The listing builds one solid part. Answer for the finished solid, in the listing's coordinates (mm). Face numbers are marked on the shaded views. A direction names the side the tool comes from. Give positions to 0.01 mm unless a question says otherwise; leave off trailing zeros. Loops run counter-clockwise (first coordinate to the right, second up) from the corner with the lowest first, then second, coordinate; pieces in that order, holes last. Notation, with made-up numbers: (-28.5, -20.5) - (-21.5, -20.5) arc R25 cw to (-21.5, 15.5) - close; hole circle Ø2 at (16.25, -6). An arc over 180 degrees is marked (long way). Answer as CSV lines item,"result". Start each with the question number.
1) A cutting plane is placed at A-A (z = 0). Determine the outline of the cut face in (x, y).
2) For the marked faces 4 and 5, determine the directions among +Z, -Z, +X, -X, +Y, -Y from which every point of the face is accessible in a straight line to the end or side of a thin tool.
3) A cutting plane is placed at D-D (x = 6.5). Determine the outline of the cut face in (y, z).
4) Find the intervals of material crossed by line 1 along Z through (x, y) = (-5.75, 8.25); line 2 along Z through (x, y) = (0, 6), in increasing order.
5) Flat-ended cylindrical pins translate along their axes: pin 1 (0.5 mm diameter, centred on y = 9, z = -7.5, fed in from -X); pin 2 (1.5 mm diameter, centred on x = -1.5, y = 8, fed in from +Z); pin 3 (0.6 mm diameter, centred on x = 0.5, z = -9, fed in from +Y); pin 4 (11 mm diameter, centred on x = 0, z = 0, fed in from +Y). Find the tip coordinate at first contact, or state that the pin passes through.
6) A cutting plane is placed at B-B (x = 0). Determine the outline of the cut face in (y, z).
7) For a pull along X with two mould halves and no side action, classify the marked faces 1, 2 and 3 as pulls with the +X half, pulls with the -X half, needs draft (parallel to the pull), parting line crosses it, or undercut.
```python
from build123d import *

# Parameters (mm, degrees)
SKETCH1_R           = 9.2
BOSS_EXTRUDE1_DEPTH = 8.2
BOSS_EXTRUDE2_DEPTH = 1.8


with BuildPart() as part:
    # Sketch1 → Boss-Extrude1 (new body)
    with BuildSketch(Plane(origin=(0, 0, 0), x_dir=(1, 0, 0), z_dir=(0, 1, 0))):
        Polygon((-10.1, 10.1), (-7, 10.1), (-7.5, 8.7), (-4.5, 8.7), (-5, 10.1), (5, 10.1), (4.5, 8.7), (7.5, 8.7), (7, 10.1), (10.1, 10.1), (10.1, 6.5), (10.1, 4.5), (10.1, -4.5), (10.1, -6.5), (10.1, -10.1), (7, -10.1), (7.5, -11.5), (4.5, -11.5), (5, -10.1), (-5, -10.1), (-4.5, -11.5), (-7.5, -11.5), (-7, -10.1), (-10.1, -10.1), (-10.1, -6.5), (-11.5, -7), (-11.5, -4), (-10.1, -4.5), (-10.1, 4.5), (-11.5, 4), (-11.5, 7), (-10.1, 6.5), align=None)
        with Locations(Location((0, 0, 0), (0, 0, 270))):
            Circle(SKETCH1_R, mode=Mode.SUBTRACT)
    extrude(amount=BOSS_EXTRUDE1_DEPTH)

    # Sketch2 → Boss-Extrude2 (add)
    with BuildSketch(Plane(origin=(0, 8.2, 0), x_dir=(1, 0, 0), z_dir=(0, 1, 0))):
        with BuildLine():
            Line((-4.1, 10.1), (-4.1, 5.1))
            ThreePointArc((-4.1, 5.1), (-4.392893219, 4.392893219), (-5.1, 4.1))
            Line((-5.1, 4.1), (-10.1, 4.1))
            Line((-10.1, 4.1), (-10.1, 10.1))
            Line((-10.1, 10.1), (-4.1, 10.1))
        make_face()
        with BuildLine():
            Line((10.1, 4.1), (10.1, 10.1))
            Line((10.1, 10.1), (4.1, 10.1))
            Line((4.1, 10.1), (4.1, 5.1))
            ThreePointArc((4.1, 5.1), (4.392893219, 4.392893219), (5.1, 4.1))
            Line((5.1, 4.1), (10.1, 4.1))
        make_face()
        with BuildLine():
            Line((4.1, -10.1), (4.1, -5.1))
            ThreePointArc((4.1, -5.1), (4.392893219, -4.392893219), (5.1, -4.1))
            Line((5.1, -4.1), (10.1, -4.1))
            Line((10.1, -4.1), (10.1, -10.1))
            Line((10.1, -10.1), (4.1, -10.1))
        make_face()
        with BuildLine():
            Line((-10.1, -4.1), (-10.1, -10.1))
            Line((-10.1, -10.1), (-4.1, -10.1))
            Line((-4.1, -10.1), (-4.1, -5.1))
            ThreePointArc((-4.1, -5.1), (-4.392893219, -4.392893219), (-5.1, -4.1))
            Line((-5.1, -4.1), (-10.1, -4.1))
        make_face()
    extrude(amount=BOSS_EXTRUDE2_DEPTH)


solid = part.part
```
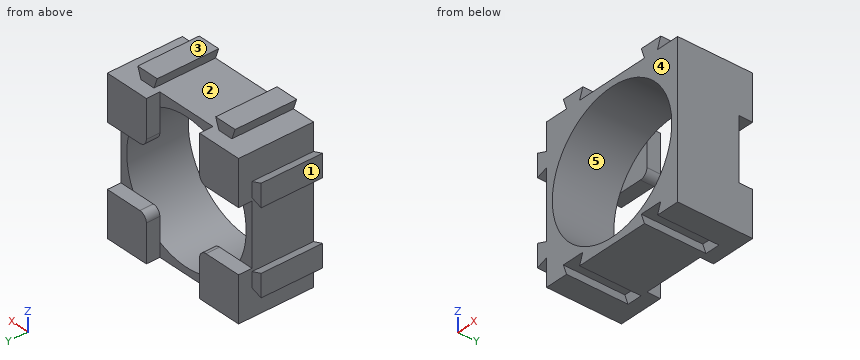
Ans:
1,outline,"(-10.1, 0) - (-9.2, 0) - (-9.2, 8.2) - (-10.1, 8.2) - close; (9.2, 0) - (10.1, 0) - (10.1, 8.2) - (9.2, 8.2) - close"
2,face 4,"+Z, -Z, +X, -X, -Y"
2,face 5,"-Y"
3,outline,"(0, -8.7) - (8.2, -8.7) - (8.2, -10.1) - (10, -10.1) - (10, -4.1) - (8.2, -4.1) - (8.2, -6.51) - (0, -6.51) - close; (0, 6.51) - (8.2, 6.51) - (8.2, 4.1) - (10, 4.1) - (10, 10.1) - (8.2, 10.1) - (8.2, 11.5) - (0, 11.5) - close"
4,line 1,"-10.1 to -4.1, 4.1 to 10.1"
4,line 2,"-10.1 to -9.2, 9.2 to 10.1"
5,pin 1,"x = -10.1"
5,pin 2,"z = 10.1"
5,pin 3,"y = 8.2"
5,pin 4,"through"
6,outline,"(0, -10.1) - (8.2, -10.1) - (8.2, -9.2) - (0, -9.2) - close; (0, 9.2) - (8.2, 9.2) - (8.2, 10.1) - (0, 10.1) - close"
7,face 1,"pulls with the -X half"
7,face 2,"undercut"
7,face 3,"needs draft"
